For this review, use the dimensioned drawing (mm, ordinates from the lowest corner) and the shaded views. Coordinates: 2 decimals unless noted, no trailing zeros. Write each loop counter-clockwise with the first axis right and the second up, starting at its lowest first coordinate (ties: lowest second). Pieces come first, ordered by that corner, then holes.
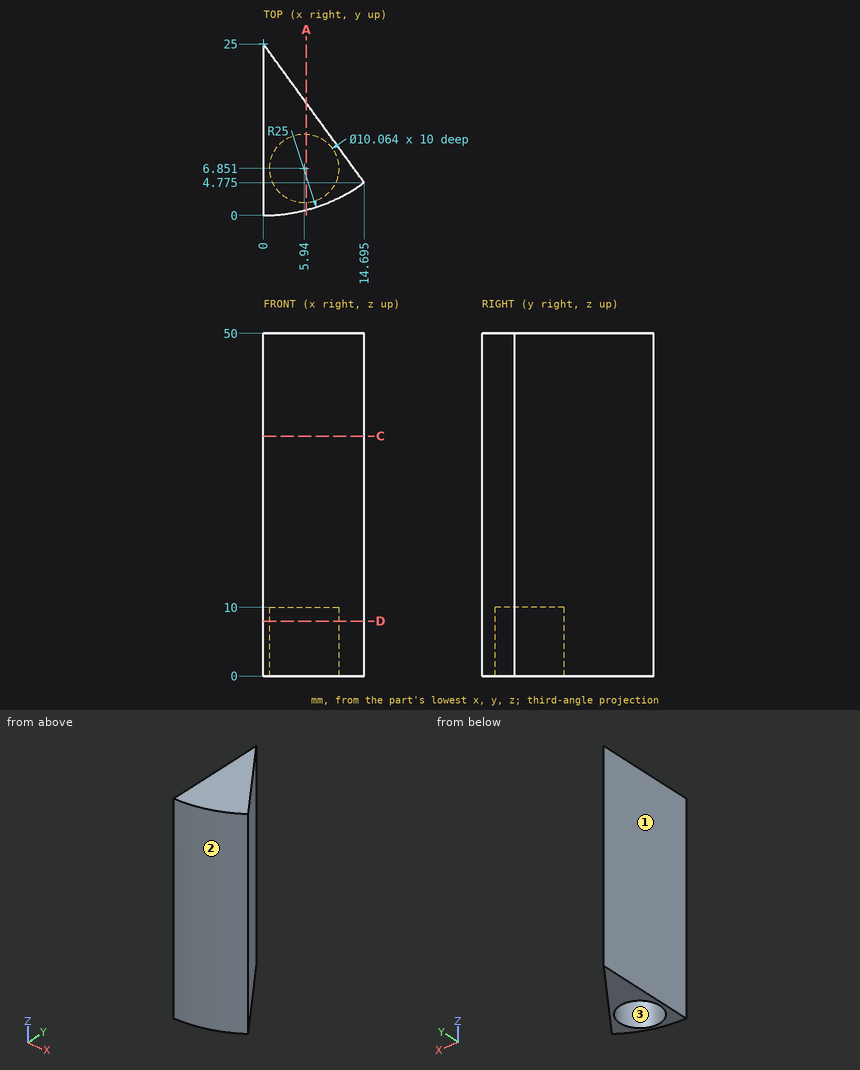
Item 1: Take a section at D-D, the plane z = 8. Write out the cut boundary in (x, y) (1 decimal), plus the area to 3 significant figures.
Solved:
outline: (0, 0) arc R25 ccw to (14.7, 4.8) - (0, 25) - close; hole circle Ø10.1 at (5.9, 6.9)
area: 117 mm2
Item 2: Mouldability with a two-part tool opening along X and no side actions: class the marked faces 1, 2 and 3 as pulls with the +X half, pulls with the -X half, needs draft (parallel to the pull), parting line crosses it, or undercut.
Solved:
face 1: pulls with the -X half
face 2: pulls with the +X half
face 3: undercut
Item 3: Take a section at A-A, the plane x = 6.25. Write out the cut boundary in (y, z), plus the area to 3 significant figures.
Solved:
outline: (0.79, 0) - (1.83, 0) - (1.83, 10) - (11.87, 10) - (11.87, 0) - (16.4, 0) - (16.4, 50) - (0.79, 50) - close
area: 680 mm2
Item 4: Take a section at C-C, the plane z = 35. Write out the cut boundary in (x, y) (1 decimal).
Solved:
outline: (0, 0) arc R25 ccw to (14.7, 4.8) - (0, 25) - close
Item 5: For pin 1 (8 mm diameter, centred on y = 8, z = 35.5, fed in from +X) (1 decimal); pin 2 (1.5 mm diameter, centred on x = 2.5, z = 5, fed in from -Y); pin 3 (8 mm diameter, centred on y = 12.5, z = 24.5, fed in from +X), all flat-tipped, find the tip position at first contact; note any pin that passes through.
Solved:
pin 1: stops at x = 14.7
pin 2: stops at y = 0.06
pin 3: stops at x = 11.99
Item 6: To check wall thickness, follow line 1 along Z through (x, y) = (5.5, 11); line 2 along Y through (x, z) = (7, 4) (1 decimal); line 3 along X through (y, z) = (11.25, 25). State the ranges of each line that lie inside material, in increasing order.
Solved:
line 1: z = 10 to 50
line 2: y = 1 to 1.9, 11.8 to 15.4
line 3: x = 0 to 9.99
